Geometry: see drawing. Coordinates: mm, zero at the bounding-box minimum. Coordinates: 2 decimals unless noted, no trailing zeros. Loops run counter-clockwise (first coordinate to the right, second up) from the corner with the lowest first, then second, coordinate; pieces in that order, holes last. Notation, with made-up numbers: (-27, -3.75) - (-23, -3.75) arc R34 cw to (-23, 29.25) - close; hole circle Ø2 at (28.25, 2.25). An arc over 180 degrees is marked (long way). Use a Markdown table: item, result. Add a question column.
1. Ray query, L1, parallel to Y at x = 26, z = 2.45; L2, parallel to X at y = 139, z = 1.1. Return the intervals inside material, ascending. Write a range as [from, to].
2. Contact query for flat-ended pins moving along their axis: P1, Ø0.9, axis at y = 198.5, z = 1, coming from the +X side; P2, Ø1.5, axis at y = 14, z = 1.5, coming from the -X side; P3, Ø1.5, axis at x = 80.5, z = 2, coming from the +Y side. Output: stop coordinate, or through.
3. Section query A-A on y = 72. Return the cut outline in (x, z), then the cut area to 3 significant figures.
4. Section query B-B on x = 39. Return the cut outline in (y, z).
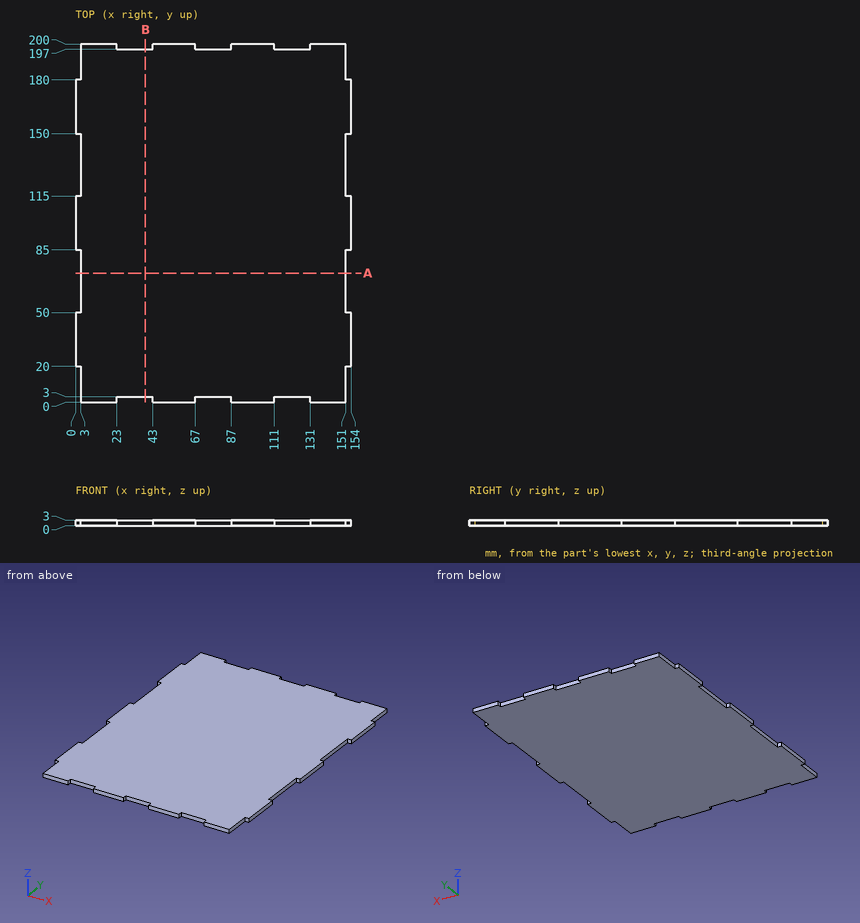
Resolved:
| question | item | result |
|---|---|---|
| 1 | L1 | [3, 197] |
| 1 | L2 | [3, 151] |
| 2 | P1 | x = 151 |
| 2 | P2 | x = 3 |
| 2 | P3 | y = 197 |
| 3 | outline | (3, 0) - (151, 0) - (151, 3) - (3, 3) - close |
| 3 | area | 444 mm² |
| 4 | outline | (3, 0) - (197, 0) - (197, 3) - (3, 3) - close |
